```python
from build123d import *

# Parameters (mm, degrees)
SKETCH1_W           = 9
SKETCH1_H           = 9
BOSS_EXTRUDE1_DEPTH = 104
SKETCH2_W           = 3
SKETCH2_H           = 6
BOSS_EXTRUDE2_DEPTH = 4.5


with BuildPart() as part:
    # Sketch1 → Boss-Extrude1 (new body, symmetric)
    with BuildSketch(Plane.XY):
        Rectangle(SKETCH1_W, SKETCH1_H)
    extrude(amount=BOSS_EXTRUDE1_DEPTH, both=True)

    # Sketch2 → Boss-Extrude2 (add, symmetric)
    with BuildSketch(Plane(origin=(0, 0, 0), x_dir=(1, 0, 0), z_dir=(0, 1, 0))):
        with Locations((-6, -83.825)):
            Rectangle(SKETCH2_W, SKETCH2_H)
        with Locations((6, -83.825)):
            Rectangle(SKETCH2_W, SKETCH2_H)
        with Locations((6, 83.825)):
            Rectangle(SKETCH2_W, SKETCH2_H)
        with Locations((-6, 83.825)):
            Rectangle(SKETCH2_W, SKETCH2_H)
    extrude(amount=BOSS_EXTRUDE2_DEPTH, both=True)


solid = part.part
```
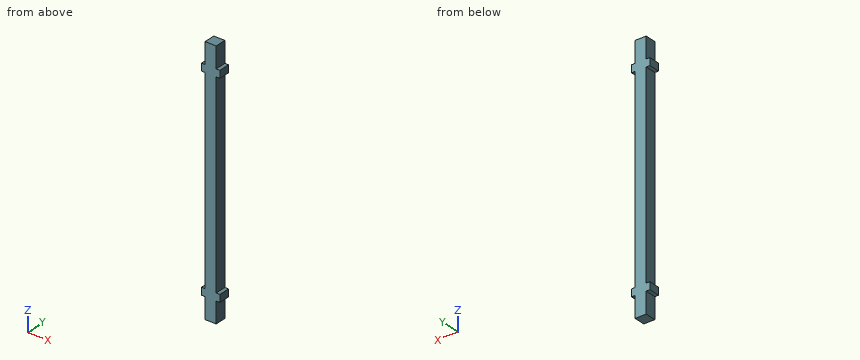
Check sheet for the modelled part. Datum: model origin and axes. Units: mm. Round coordinates to 2 decimals unless told otherwise and drop trailing zeros. Loops run counter-clockwise (first coordinate to the right, second up) from the corner with the lowest first, then second, coordinate; pieces in that order, holes last. Notation, with made-up numbers: (1.25, 34.5) - (25.25, 34.5) arc R23 cw to (25.25, 67.5) - close; hole circle Ø9 at (50.25, 5.5). An arc over 180 degrees is marked (long way). Write item = value, one per line. Start each with the question number.
Q1. Section check A-A (y = 2.75). Record the boundary of the cut face in (x, z) (3 decimals), plus the area to 3 significant figures.
Q2. Depth check by flat-ended pin: P1, Ø2.5, axis at x = -6, y = 0.5, coming from the +Z side (3 decimals); P2, Ø2.5, axis at y = -0.5, z = -40, coming from the +X side; P3, Ø1.5, axis at x = -6.5, y = 0.5, coming from the -Z side (3 decimals). Enter the tip coordinate at first touch or a pass-through.
Q3. Section check B-B (z = -35). Record the boundary of the cut face in (x, y), plus the area to 3 significant figures.
Q4. Thickness scan on L1, parallel to X at y = 0.25, z = 22.5. Record the ranges inside material, lowest first.
Derived:
q1.outline = (-7.5, -86.825) - (-4.5, -86.825) - (-4.5, -104) - (4.5, -104) - (4.5, -86.825) - (7.5, -86.825) - (7.5, -80.825) - (4.5, -80.825) - (4.5, 80.825) - (7.5, 80.825) - (7.5, 86.825) - (4.5, 86.825) - (4.5, 104) - (-4.5, 104) - (-4.5, 86.825) - (-7.5, 86.825) - (-7.5, 80.825) - (-4.5, 80.825) - (-4.5, -80.825) - (-7.5, -80.825) - close
q1.area = 1,940 mm^2
q2.P1 = 86.825
q2.P2 = 4.5
q2.P3 = -86.825
q3.outline = (-4.5, -4.5) - (4.5, -4.5) - (4.5, 4.5) - (-4.5, 4.5) - close
q3.area = 81.0 mm^2
q4.L1 = -4.5 to 4.5
